from build123d import *

# Parameters (mm, degrees)
THDSCHPAT_COUNT = 16
THDSCHPAT_PITCH = 1.27


with BuildPart() as part:
    # BodySke → Base-Revolve (revolve)
    with BuildSketch(Plane.XY):
        with BuildLine():
            Line((0, 0), (60.579, 0))
            Line((60.579, 0), (60.579, 3.175))
            Line((60.579, 3.175), (3.8354, 3.175))
            ThreePointArc((3.8354, 3.175), (3.548031804, 3.294031804), (3.429, 3.5814))
            Line((3.429, 3.5814), (3.429, 7.3533))
            Line((3.429, 7.3533), (3.302, 7.3533))
            ThreePointArc((3.302, 7.3533), (0.863382865, 4.030329543), (0, 0))
        make_face()
    revolve(axis=Axis((0, 0, 0), (1, 0, 0)))

    # ThdSchSke → ThreadSchematic (revolve, cut)
    with BuildSketch(Plane.XY):
        Polygon((41.529, -2.41935), (40.999888174, -3.175), (40.999888174, -3.96875), (42.058111826, -3.96875), (42.058111826, -3.175), align=None)
    threadschematic = revolve(axis=Axis((-3.175, 0, 0), (1, 0, 0)), mode=Mode.SUBTRACT)

    # ThdSchPat: ThreadSchematic ×16
    with Locations(*[(i * THDSCHPAT_PITCH, 0, 0) for i in range(1, THDSCHPAT_COUNT)]):
        add(threadschematic, mode=Mode.SUBTRACT)


solid = part.part
The listing builds one solid part. Answer for the finished solid, in the listing's coordinates (mm). Give positions to 0.01 mm unless a question says otherwise; leave off trailing zeros. Order: outer loops, then holes, each group sorted by start corner. A loop starts at its lowest first (then second) coordinate and runs counter-clockwise, first axis right, second up. Notation, with made-up numbers: (20, -25) - (78, -25) arc R16 cw to (78, -6) - close; hole circle Ø8 at (9, 39). An arc over 180 degrees is marked (long way). One line per item, written item: value. Start each with the question number.
1) Find the intervals of material crossed by L1, parallel to Z at x = 55, y = 2; L2, parallel to Z at x = 22, y = 0 (3 decimals); L3, parallel to X at y = -1, z = -4, in increasing order.
2) A cutting plane is placed at B-B on z = 6.5. Give the vertices of the cut face in (x, y).
3) Given pin 1 Ø6 at (x, z) = (19.5, 0.5) entering from -Y (3 decimals); pin 2 Ø1.5 at (x, z) = (49, -4) entering from -Y; pin 3 Ø1.5 at (x, z) = (41, -2) entering from -Y; pin 4 Ø6 at (x, y) = (46.5, -4) entering from +Z, each flat-ended and moving along its own axis, determine where each tip first touches the part or whether it passes through.
4) A cutting plane is placed at A-A on x = 39. Give the vertices of the cut face in (y, z) (3 decimals).
Answer sheet:
1. L1: z = -2.41 to 2.41
1. L2: z = -3.175 to 3.175
1. L3: x = 0.91 to 3.43
2. outline: (3.3, -3.44) - (3.43, -3.44) - (3.43, 3.44) - (3.3, 3.44) arc R7.39 ccw to start
3. pin 1: stops at y = -3.175
3. pin 2: passes through
3. pin 3: stops at y = -2.92
3. pin 4: stops at z = 3
4. outline: circle Ø6.35 at (0, 0)
